Geometry: final body of the model. Coordinates: model frame, mm. Coordinates: 2 decimals unless noted, no trailing zeros. Order: outer loops, then holes, each group sorted by start corner. A loop starts at its lowest first (then second) coordinate and runs counter-clockwise, first axis right, second up. Notation, with made-up numbers: (-11, -10.75) -> (20, -10.75) arc R20 ccw to (20, 9.25) -> close; hole circle Ø1 at (-32.75, -18). An arc over 180 degrees is marked (long way). Use one line per item in the form item = value.
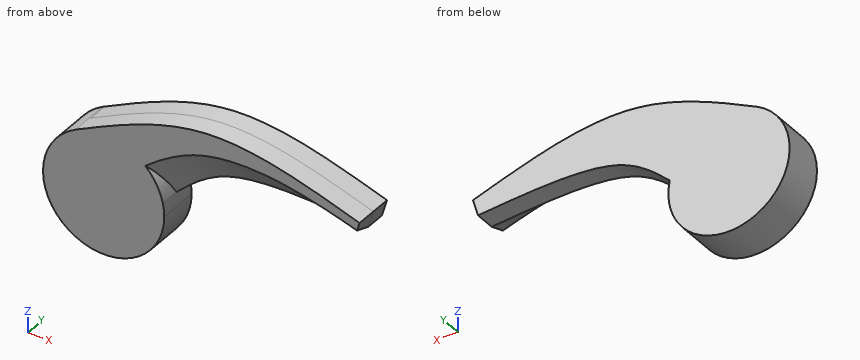
```python
from build123d import *

# Parameters (mm, degrees)
F6_DEPTH = 10
F7_DEPTH = 20


# Not quite as in the source:
# - the dataset's text gives a spline's control points without its knots; the knots are read off the source's solid


with BuildPart() as f5:
    # F3 (on offset) → F5 section 0
    with BuildSketch(Plane.XZ.offset(10)):
        with BuildLine():
            ThreePointArc((-75.5787535417, 16.7525420321), (-74.2842309522, -36.7668523877), (-32.5165676908, -3.2785906609))
            add(Edge.make_bspline(
                [(-32.5165676908, -3.2785906609), (-25.0186225888, 3.7525831829), (-6.6027990329, 21.0474968683), (36.4369216658, 17.5617465832), (61.9822815061, 15.4927987605)],
                knots=[0, 0, 0, 0, 0.406452044, 1, 1, 1, 1], degree=3))
            Line((61.9822815061, 15.4927987605), (64.4333958626, 23.9602774382))
            add(Edge.make_bspline(
                [(-75.5787535417, 16.7525420321), (-54.628951456, 27.285399841), (-11.406645731, 48.9685404457), (38.647869417, 32.4670255034), (64.4333958626, 23.9602774382)],
                knots=[0, 0, 0, 0, 0.4849009259, 1, 1, 1, 1], degree=3))
        make_face()
    # F4 (on offset) → F5 section 1
    with BuildSketch(Plane.XZ.offset(20)):
        with BuildLine():
            add(Edge.make_bspline(
                [(-75.5787535417, 16.7525420321), (-54.628951456, 27.285399841), (-11.406645731, 48.9685404457), (38.647869417, 32.4670255034), (64.4333958626, 23.9602774382)],
                knots=[0, 0, 0, 0, 0.4849009259, 1, 1, 1, 1], degree=3))
            ThreePointArc((-75.5787535417, 16.7525420321), (-65.7534042192, -39.2752402765), (-41.1793711539, 12.0255080478))
            add(Edge.make_bspline(
                [(-41.1793711539, 12.0255080478), (-25.2502910967, 24.6854926251), (-0.0760708598, 33.9443363857), (36.1576432322, 28.3926800744), (63.2078386843, 19.7265380993)],
                knots=[0, 0, 0, 0, 0.4558632428, 1, 1, 1, 1], degree=3))
            Line((63.2078386843, 19.7265380993), (64.4333958626, 23.9602774382))
        make_face()
    loft()

    # F0 (on Front) → F6 (join)
    with BuildSketch(Plane.XZ):
        with BuildLine():
            ThreePointArc((-74.6210650057, 17.2339850929), (-48.6067992872, 17.1628264037), (-32.5165676908, -3.2785906609))
            add(Edge.make_bspline(
                [(-32.5165676908, -3.2785906609), (-25.0186225888, 3.7525831829), (-6.6027990329, 21.0474968683), (36.4369216658, 17.5617465832), (61.9822815061, 15.4927987605)],
                knots=[0, 0, 0, 0, 0.406452044, 1, 1, 1, 1], degree=3))
            Line((61.9822815061, 15.4927987605), (64.4333958626, 23.9602774382))
            add(Edge.make_bspline(
                [(-74.6210650057, 17.2339850929), (-53.9898610909, 27.6037376874), (-11.0368055784, 48.8466149254), (38.647869417, 32.4670255034), (64.4333958626, 23.9602774382)],
                knots=[0.0073887471, 0.0073887471, 0.0073887471, 0.0073887471, 0.4849009259, 1, 1, 1, 1], degree=3))
        make_face()
    extrude(amount=F6_DEPTH)

    # F0 (on Front) → F7 (join)
    with BuildSketch(Plane.XZ):
        with BuildLine():
            ThreePointArc((-75.5787535417, 16.7525420321), (-77.1329137918, -35.2493874652), (-31.8209869176, -9.6868099645))
            ThreePointArc((-31.8209869176, -9.6868099645), (-31.9953913254, -6.4638801151), (-32.5165676908, -3.2785906609))
            ThreePointArc((-32.5165676908, -3.2785906609), (-48.6067992872, 17.1628264037), (-74.6210650057, 17.2339850929))
            add(Edge.make_bspline(
                [(-75.5787535417, 16.7525420321), (-75.2595279418, 16.9130379566), (-74.940300314, 17.0735295431), (-74.6210650057, 17.2339850929)],
                knots=[0, 0, 0, 0, 0.0073887471, 0.0073887471, 0.0073887471, 0.0073887471], degree=3))
        make_face()
    extrude(amount=F7_DEPTH)


solid = f5.part
```
1) Contact query for flat-ended pins moving along their axis: P1, Ø12, axis at x = 40.5, y = -4.5, coming from the +Z side; P2, Ø10, axis at x = -32.5, y = -14, coming from the +Z side; P3, Ø4, axis at y = -11, z = 5.5, coming from the -X side. Output: stop coordinate, or through.
Results found:
P1 = 33.27
P2 = 36.7
P3 = -88.49
2) Material intervals for probe 1 along X at (y, z) = (-7.5, -8.5); probe 2 along X at (y, z) = (-6.75, -25.5); probe 3 along Z at (x, y) = (23, -5.25), sorted ascending. Write a range as from..to.
Results found:
probe_1 = -91.53..-31.84
probe_2 = -87.02..-36.35
probe_3 = 17.69..36.13
3) Section A-A, the plane z = -20. Output: boundary loops of the cut face in (x, y), and give its area (3 significant figures).
Results found:
outline = (-89.72, -20) -> (-33.66, -20) -> (-33.66, 0) -> (-89.72, 0) -> close
area = 1,120 mm2
